Autodesk Inventor part; units mm, degrees
ref_plane "YZ Plane" through (0, 0, 0) normal (1, 0, 0) x (0, 1, 0)
ref_plane "XZ Plane" through (0, 0, 0) normal (0, 1, 0) x (-1, 0, 0)
ref_plane "XY Plane" through (0, 0, 0) normal (0, 0, 1) x (1, 0, 0)
sketch "Sketch1" plane through (0, 0, 0) normal (0, 1, 0) x (-1, 0, 0)
  line L0 (6, 8) -> (-6, 8)
  line L1 (-8, 6) -> (-8, -6)
  line L2 (-6, -8) -> (6, -8)
  line L3 (8, -6) -> (8, 6)
  arc A0 (8, 6) -> (6, 8) centre (6, 6) ccw
  arc A1 (-6, 8) -> (-8, 6) centre (-6, 6) ccw
  arc A2 (-8, -6) -> (-6, -8) centre (-6, -6) ccw
  arc A3 (6, -8) -> (8, -6) centre (6, -6) ccw
  point P0 (0, 0)
  point P1 (8, 8)
  point P2 (-8, 8)
  point P3 (8, -8)
  dimension "d0" = 16
  dimension "d1" = 16
  dimension "d2" = 8
  dimension "d3" = 8
  dimension "d4" = 2
extrude "Extrusion1" add sketch "Sketch1" along normal blind 50
sketch "Sketch2" plane through (0, 0, 0) normal (0, -1, 0) x (1, 0, 0)
  line L0 (-6, 5.875) -> (-6, 3.125) construction
  line L1 (-7.375, 5.875) -> (-7.375, 3.125)
  line L2 (-4.625, 3.125) -> (-4.625, 5.875)
  arc A0 (-4.625, 5.875) -> (-7.375, 5.875) centre (-6, 5.875) ccw
  arc A1 (-7.375, 3.125) -> (-4.625, 3.125) centre (-6, 3.125) ccw
  line L3 (6, -3.125) -> (6, -5.875) construction
  line L4 (4.625, -3.125) -> (4.625, -5.875)
  line L5 (7.375, -5.875) -> (7.375, -3.125)
  arc A2 (7.375, -3.125) -> (4.625, -3.125) centre (6, -3.125) ccw
  arc A3 (4.625, -5.875) -> (7.375, -5.875) centre (6, -5.875) ccw
  point P0 (0, 0)
  point P1 (0, 0)
  point P2 (-6, 4.5)
  point P3 (6, -4.5)
  dimension "d7" = 2.75
  dimension "d8" = 12
  dimension "d9" = 6
  dimension "d10" = 9
  dimension "d11" = 4.5
  dimension "d12" = 2.75
  dimension "d13" = 2.75
  dimension "d14" = 2.75
extrude "Extrusion2" cut sketch "Sketch2" against normal blind 2.5
hole "Hole1" at (0, 0, 0) direction (0, 1, 0) diameter 6.756 end through all
sketch "Sketch3" plane through (0, 50, 0) normal (0, 1, 0) x (1, 0, 0)
  line L0 (-6, 1.5) -> (-6, -1.5) construction
  line L1 (-6.6, 1.5) -> (-6.6, -1.5)
  line L2 (-5.4, -1.5) -> (-5.4, 1.5)
  arc A0 (-5.4, 1.5) -> (-6.6, 1.5) centre (-6, 1.5) ccw
  arc A1 (-6.6, -1.5) -> (-5.4, -1.5) centre (-6, -1.5) ccw
  line L3 (6, 1.5) -> (6, -1.5) construction
  line L4 (5.4, 1.5) -> (5.4, -1.5)
  line L5 (6.6, -1.5) -> (6.6, 1.5)
  arc A2 (6.6, 1.5) -> (5.4, 1.5) centre (6, 1.5) ccw
  arc A3 (5.4, -1.5) -> (6.6, -1.5) centre (6, -1.5) ccw
  line L6 (-6, 0) -> (6, 0) construction
  line L7 (6, 8) -> (-6, 8)
  point P0 (0, 0)
  dimension "d25" = 0.6
  dimension "d26" = 0.6
  dimension "d27" = 3
  dimension "d29" = 0
  dimension "d30" = 12
  dimension "d31" = 6
  dimension "d32" = 3
extrude "Extrusion3" add sketch "Sketch3" along normal blind 1.5
equation "\"d12\" = d7"
equation "\"d13\" = d7"
equation "\"d14\" = d7"
equation "\"d26\" = d25"
equation "\"d27\" = d32"
properties part number "Camera Mount 30mm"
Geometry check sheet. Reference: the model listing, model coordinates, mm. A direction names the side the tool comes from. Coordinates: 2 decimals unless noted, no trailing zeros. Order: outer loops, then holes, each group sorted by start corner. A loop starts at its lowest first (then second) coordinate and runs counter-clockwise, first axis right, second up. Notation, with made-up numbers: M 86,19.5 L 143,19.5 A37 cw 143,58.5 Z; hole C 51,79.5 d5. An arc over 180 degrees is marked long. Answer as a JSON object with one key per item and string values.
Q1. Depth check by flat-ended pin: pin 1 Ø1.6 at (y, z) = (50.5, -0.5) entering from +X; pin 2 Ø5 at (x, z) = (-2, 2) entering from +Y; pin 3 Ø1.4 at (x, z) = (-5.5, 3) entering from -Y; pin 4 Ø1.2 at (y, z) = (51, -0.5) entering from +X. Enter the tip coordinate at first touch or a pass-through.
Results are:
{"pin 1": "stops at x = 8", "pin 2": "stops at y = 50", "pin 3": "stops at y = 2.5", "pin 4": "stops at x = 6.6"}
Q2. Release check for a two-part mould opening along Z. For faces 6 (the cylindrical face through (7.43, 24.65, 7.4)), 7 (the flat face through (-4.625, 1, 4)), 8 (the flat face through (-8, 25, 0)) record: released by +Z, released by -Z, zero draft, split by the parting line, or undercut.
Results are:
{"face 6": "released by +Z", "face 7": "undercut", "face 8": "zero draft"}
Q3. Cross-section at B-B on x = 0. Record the cut outline in (y, z), and give its area (3 significant figures).
Results are:
{"outline": "M 0,-8 L 50,-8 L 50,-3.38 L 0,-3.38 Z; M 0,3.38 L 50,3.38 L 50,8 L 0,8 Z", "area": "462 mm²"}
Q4. Cross-section at A-A on y = 23. Record the cut outline in (x, z).
Results are:
{"outline": "M -8,-6 A2 ccw -6,-8 L 6,-8 A2 ccw 8,-6 L 8,6 A2 ccw 6,8 L -6,8 A2 ccw -8,6 Z; hole C 0,0 d6.76"}
Q5. Tool access check on faces 1 (the cylindrical face through (6, 50.7, -2.1)), 2 (the cylindrical face through (6, 50.7, 2.1)), 3 (the flat face through (8, 25, 0)), 4 (the cylindrical face through (-5.97, 1.23, 7.25)), 5 (the flat face through (-6.6, 51, 0)). Record the directions out of +Z, -Z, +X, -X, +Y, -Y that give a thin tool (end or side, any length) a straight path to the whole face; none if there is none.
Results are:
{"face 1": "-Z, +Y", "face 2": "+Z, +Y", "face 3": "+Z, -Z, +X, +Y, -Y", "face 4": "-Y", "face 5": "+Z, -Z, -X, +Y"}
Q6. Cross-section at D-D on z = -4.5. Record the cut outline in (x, y) (3 decimals), and give its area (3 significant figures).
Results are:
{"outline": "M -8,0 L 4.625,0 L 4.625,2.5 L 7.375,2.5 L 7.375,0 L 8,0 L 8,50 L -8,50 Z", "area": "793 mm²"}
Q7. Scan lines: line 1 (X direction, y = 26.5, z = 0); line 2 (Y direction, x = -0.75, z = -4.5); line 3 (X direction, y = 10, z = -2.75). Record each from-to range of solid material in increasing order.
Results are:
{"line 1": "x = -8 to -3.38, 3.38 to 8", "line 2": "y = 0 to 50", "line 3": "x = -8 to -1.96, 1.96 to 8"}
Q8. Cross-section at C-C on z = 0. Record the cut outline in (x, y).
Results are:
{"outline": "M -8,0 L -3.38,0 L -3.38,50 L -5.4,50 L -5.4,51.5 L -6.6,51.5 L -6.6,50 L -8,50 Z; M 3.38,0 L 8,0 L 8,50 L 6.6,50 L 6.6,51.5 L 5.4,51.5 L 5.4,50 L 3.38,50 Z"}
